```python
from build123d import *

# Parameters (mm, degrees)
F1_DEPTH      = 10
F1_DEPTH_BACK = 5


with BuildPart() as f1:
    # F0 (on Top) → F1 (new body, two sides)
    with BuildSketch(Plane.XY) as f1_sk:
        Polygon((-57, -29), (-57, 46), (-58, 46), (-58, -29.225431), (-48.132079, -50), (48.132079, -50), (58, -29.225431), (58, 46), (57, 46), (57, -29), (47.5, -49), (-47.5, -49), align=None)
    extrude(amount=F1_DEPTH)
    extrude(f1_sk.sketch, amount=-F1_DEPTH_BACK)


solid = f1.part
```
Check sheet for the modelled part. Datum: model origin and axes. Units: mm. A direction names the side the tool comes from. Give positions to 0.01 mm unless a question says otherwise; leave off trailing zeros. Write each loop counter-clockwise with the first axis right and the second up, starting at its lowest first coordinate (ties: lowest second). Pieces come first, ordered by that corner, then holes. Notation, with made-up numbers: (-29.75, 63.5) - (18.25, 63.5) arc R5 ccw to (18.25, 71.5) - close; hole circle Ø8 at (-34.75, 12). An arc over 180 degrees is marked (long way). Answer as a JSON object with one key per item and string values. Group by question number.
1) Thickness scan on probe 1 along X at (y, z) = (-22.5, 2); probe 2 along Y at (x, z) = (-21, -1.25); probe 3 along X at (y, z) = (-44, 1.75) (3 decimals). Record the ranges inside material, lowest first. Write a range as from..to.
2) Sectioned sample at C-C (x = -38). Record the cut outline in (y, z).
3) Depth check by flat-ended pin: P1, Ø2, axis at x = 8.5, z = 1, coming from the +Y side; P2, Ø6, axis at y = -38.5, z = 4.5, coming from the -X side. Enter the tip coordinate at first touch or a pass-through.
4) Sectioned sample at A-A (y = -15). Record the cut outline in (x, z).
5) Access from +Z, -Z, +X, -X, +Y, -Y to the whole of each face (thin tool, end or side, straight path). Record for faces 5 (the face through (58, 8, 3)), 6 (the face through (57, 9, 3)).
6) Release check for a two-part mould opening along X. For faces 1 (the face through (52.997, -39.758, 2.605)), 2 (the face through (-1, -50, 3)), 3 (the face through (-58, 9, 3)), 4 (the face through (52.316, -38.86, 2.605)) record: pulls with the +X half, pulls with the -X half, needs draft (parallel to the pull), parting line crosses it, or undercut.
7) Sectioned sample at D-D (y = -40.5). Record the cut outline in (x, z).
8) Sectioned sample at B-B (z = -2). Record the cut outline in (x, y).
Geometry results:
{
 "1": {"probe 1": "x = -58..-57, 57..58", "probe 2": "y = -50..-49", "probe 3": "x = -50.982..-49.875, 49.875..50.982"},
 "2": {"outline": "(-50, -5) - (-49, -5) - (-49, 10) - (-50, 10) - close"},
 "3": {"P1": "stops at y = -49", "P2": "stops at x = -55.02"},
 "4": {"outline": "(-58, -5) - (-57, -5) - (-57, 10) - (-58, 10) - close; (57, -5) - (58, -5) - (58, 10) - (57, 10) - close"},
 "5": {"face 5": "+Z, -Z, +X, +Y, -Y", "face 6": "+Z, -Z, +Y"},
 "6": {"face 1": "pulls with the +X half", "face 2": "needs draft", "face 3": "pulls with the -X half", "face 4": "undercut"},
 "7": {"outline": "(-52.64, -5) - (-51.54, -5) - (-51.54, 10) - (-52.64, 10) - close; (51.54, -5) - (52.64, -5) - (52.64, 10) - (51.54, 10) - close"},
 "8": {"outline": "(-58, -29.23) - (-48.13, -50) - (48.13, -50) - (58, -29.23) - (58, 46) - (57, 46) - (57, -29) - (47.5, -49) - (-47.5, -49) - (-57, -29) - (-57, 46) - (-58, 46) - close"}
}
